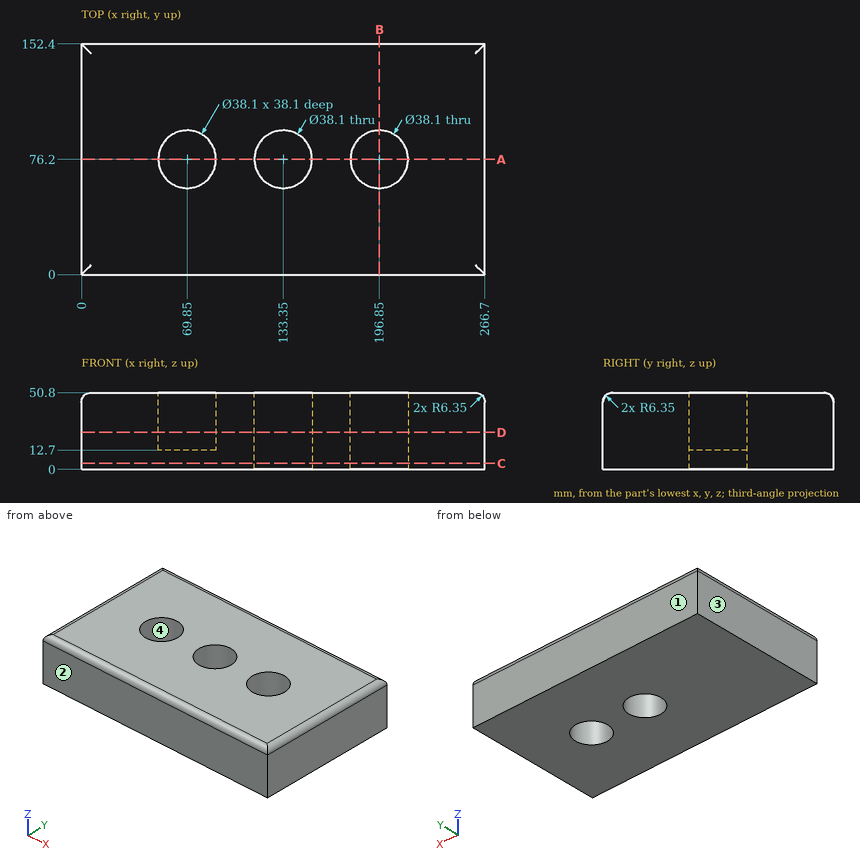
Design review of the part shown in the three views and the two pictorial views. Dimensions are in mm from the part's minimum x, y and z. Give positions to 0.01 mm unless a question says otherwise; leave off trailing zeros. Loops run counter-clockwise (first coordinate to the right, second up) from the corner with the lowest first, then second, coordinate; pieces in that order, holes last. Notation, with made-up numbers: (31.25, -23.5) -> (85.25, -23.5) arc R14 cw to (85.25, -8.5) -> close; hole circle Ø11 at (74.25, 62). An arc over 180 degrees is marked (long way). Put each result on its own line as item: value. Start each with the question number.
1. We need section A-A on y = 76.2. State the section outline as (x, z) points, then the cut area to 3 significant figures.
2. We need section D-D on z = 24.5. State the section outline as (x, y) points, then the cut area to 3 significant figures.
3. We need section B-B on x = 196.85. State the section outline as (y, z) points, then the cut area to 3 significant figures.
4. We need section C-C on z = 4. State the section outline as (x, y) points.
5. Wall thickness on probe 1 along X at (y, z) = (76, 20); probe 2 along Y at (x, z) = (133, 31); probe 3 along X at (y, z) = (92.5, 46.5): over which ranges is each line inside the solid? List them lowest first.
6. Mouldability with a two-part tool opening along Y and no side actions: class the marked faces 1, 2, 3 and 4 as released by +Y, released by -Y, zero draft, split by the parting line, or undercut.
Determined:
1. outline: (0, 0) -> (114.3, 0) -> (114.3, 50.8) -> (88.9, 50.8) -> (88.9, 12.7) -> (50.8, 12.7) -> (50.8, 50.8) -> (6.35, 50.8) arc R6.35 ccw to (0, 44.45) -> close; (152.4, 0) -> (177.8, 0) -> (177.8, 50.8) -> (152.4, 50.8) -> close; (215.9, 0) -> (266.7, 0) -> (266.7, 44.45) arc R6.35 ccw to (260.35, 50.8) -> (215.9, 50.8) -> close
1. area: 8,210 mm^2
2. outline: (0, 0) -> (266.7, 0) -> (266.7, 152.4) -> (0, 152.4) -> close; hole circle Ø38.1 at (69.85, 76.2); hole circle Ø38.1 at (133.35, 76.2); hole circle Ø38.1 at (196.85, 76.2)
2. area: 37,200 mm^2
3. outline: (0, 0) -> (57.15, 0) -> (57.15, 50.8) -> (6.35, 50.8) arc R6.35 ccw to (0, 44.45) -> close; (95.25, 0) -> (152.4, 0) -> (152.4, 44.45) arc R6.35 ccw to (146.05, 50.8) -> (95.25, 50.8) -> close
3. area: 5,790 mm^2
4. outline: (0, 0) -> (266.7, 0) -> (266.7, 152.4) -> (0, 152.4) -> close; hole circle Ø38.1 at (133.35, 76.2); hole circle Ø38.1 at (196.85, 76.2)
5. probe 1: 0 to 50.8, 88.9 to 114.3, 152.4 to 177.8, 215.9 to 266.7
5. probe 2: 0 to 57.15, 95.25 to 152.4
5. probe 3: 0.34 to 59.99, 79.71 to 123.49, 143.21 to 186.99, 206.71 to 266.36
6. face 1: released by +Y
6. face 2: released by -Y
6. face 3: zero draft
6. face 4: undercut
